The figure shows three views and two pictorial views of one solid part (mm, origin at its lowest corner). Answer the questions. Coordinates: 2 decimals unless noted, no trailing zeros. Order: outer loops, then holes, each group sorted by start corner. A loop starts at its lowest first (then second) coordinate and runs counter-clockwise, first axis right, second up.
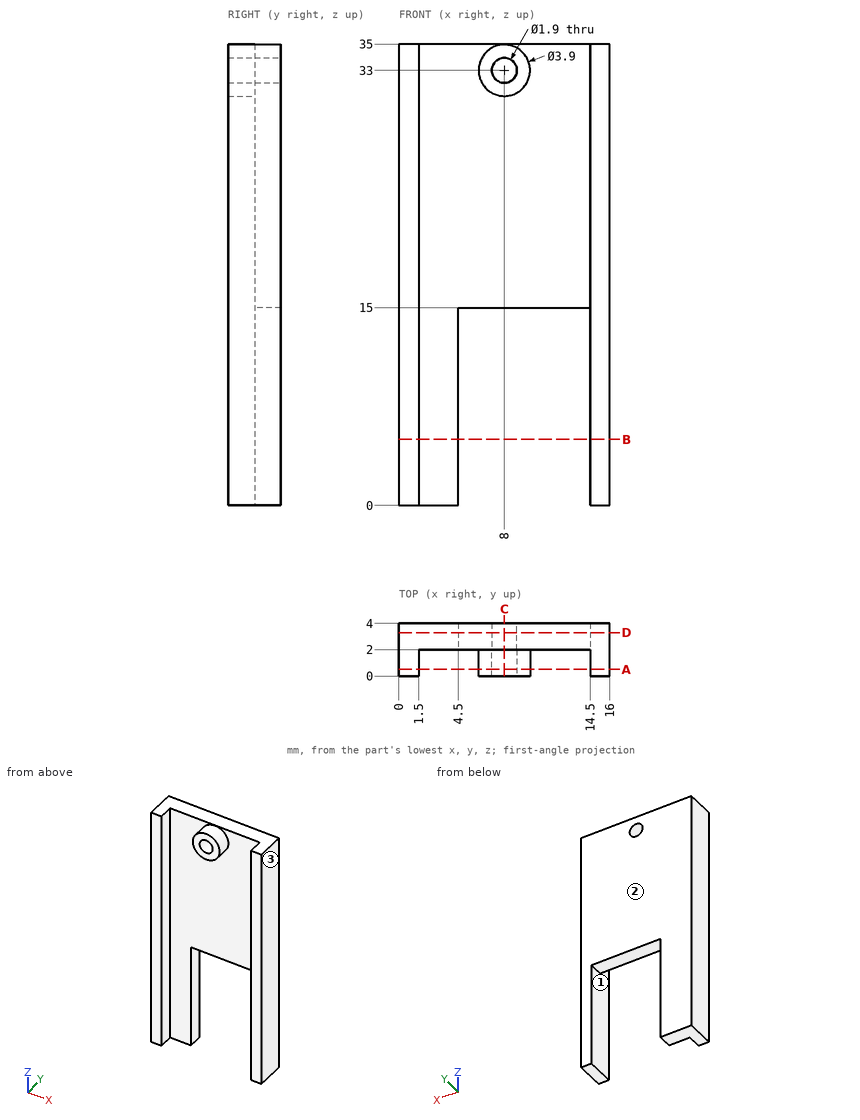
1) Each of these flat-tipped pins is pushed along its axis until it touches: P1, Ø4, axis at x = 10, z = 24.5, coming from the -Y side; P2, Ø0.6, axis at x = 10.5, y = 3, coming from the -Z side. Where does it stop, or does it pass through?
2) A cutting plane is placed at C-C, the plane x = 8. Write down the section's boundary in (y, z), plus the area to 3 significant figures.
3) The mould has two halves that part along X. Classify the marked faces 1, 2 and 3: released by +X, released by -X, zero draft, split by the parting line, or undercut.
4) A cutting plane is placed at B-B, the plane z = 5. Write down the section's boundary in (x, y).
5) A cutting plane is placed at A-A, the plane y = 0.5. Write down the section's boundary in (x, z).
6) Straight lines are drawn through the part: probe 1 along Z at (x, y) = (8, 1.55); probe 2 along X at (y, z) = (2.5, 9.5); probe 3 along X at (y, z) = (2.05, 33). For each, find the intervals that lie inside material, in ascending order.
7) A cutting plane is placed at D-D, the plane y = 3.3. Write down the section's boundary in (x, z).
Working result:
1. P1: stops at y = 2
1. P2: stops at z = 15
2. outline: (0, 31.05) - (2, 31.05) - (2, 15) - (4, 15) - (4, 32.05) - (0, 32.05) - close; (0, 33.95) - (4, 33.95) - (4, 35) - (2, 35) - (2, 34.95) - (0, 34.95) - close
2. area: 40.2 mm2
3. face 1: undercut
3. face 2: zero draft
3. face 3: released by +X
4. outline: (0, 0) - (1.5, 0) - (1.5, 2) - (4.5, 2) - (4.5, 4) - (0, 4) - close; (14.5, 0) - (16, 0) - (16, 4) - (14.5, 4) - close
5. outline: (0, 0) - (1.5, 0) - (1.5, 35) - (0, 35) - close; circle Ø3.9 at (8, 33); (14.5, 0) - (16, 0) - (16, 35) - (14.5, 35) - close; hole circle Ø1.9 at (8, 33)
6. probe 1: z = 31.05 to 32.05, 33.95 to 34.95
6. probe 2: x = 0 to 4.5, 14.5 to 16
6. probe 3: x = 0 to 7.05, 8.95 to 16
7. outline: (0, 0) - (4.5, 0) - (4.5, 15) - (14.5, 15) - (14.5, 0) - (16, 0) - (16, 35) - (0, 35) - close; hole circle Ø1.9 at (8, 33)
